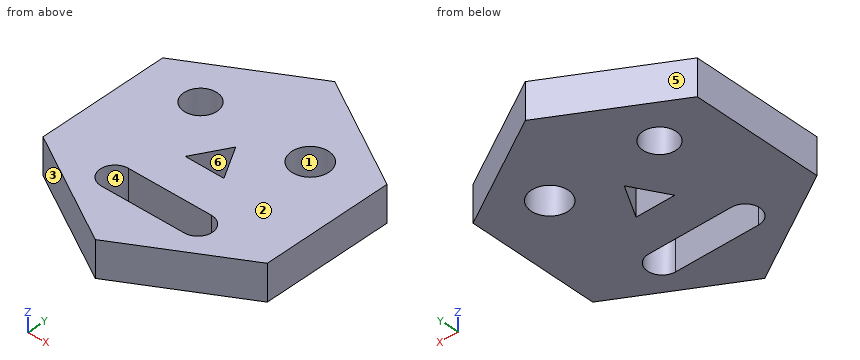
from build123d import *

# Parameters (mm, degrees)
SKETCH_R   = 4.618848
SKETCH_R_2 = 5.157962
PAD_DEPTH  = 10


with BuildPart() as part:
    # Sketch → Pad (new body)
    with BuildSketch(Plane.XY):
        Polygon((96.723577, 31.138338), (96.674117, 67.116094), (65.491737, 85.062138), (34.358817, 67.030427), (34.408277, 31.052671), (65.590657, 13.106627), align=None)
        with Locations((50.045269, 61.452663)):
            Circle(SKETCH_R, mode=Mode.SUBTRACT)
        with Locations((80.082733, 61.98597)):
            Circle(SKETCH_R_2, mode=Mode.SUBTRACT)
        with BuildLine():
            ThreePointArc((54.325382, 35.182339), (50.269895, 31.126852), (54.325382, 27.071365))
            Line((54.325382, 27.071365), (77.411652, 27.071365))
            ThreePointArc((77.411652, 27.071365), (81.467139, 31.126852), (77.411652, 35.182339))
            Line((54.325382, 35.182339), (77.411652, 35.182339))
        make_face(mode=Mode.SUBTRACT)
        Polygon((65.553779, 55.296537), (60.155022, 45.989201), (70.91479, 45.967409), align=None, mode=Mode.SUBTRACT)
    extrude(amount=PAD_DEPTH)


solid = part.part
Input: part model. Units: mm. Frame: model coordinates. Face numbers are marked on the shaded views. A direction names the side the tool comes from. Give positions to 0.01 mm unless a question says otherwise; leave off trailing zeros. Loops run counter-clockwise (first coordinate to the right, second up) from the corner with the lowest first, then second, coordinate; pieces in that order, holes last. Notation, with made-up numbers: (14.25, 69.5) -> (70.25, 69.5) arc R19 ccw to (70.25, 82.5) -> close; hole circle Ø5 at (-34.75, 71.25). An arc over 180 degrees is marked (long way). Answer as a JSON object with one key per item and string values. Group by question number.
Item 1: Cut plane D-D, the plane y = 58. Return the cut outline in (x, z), and give its area (3 significant figures).
Item 2: Cut plane B-B, the plane x = 58. Return the cut outline in (y, z).
Item 3: Line query: probe 1 along Y at (x, z) = (80, 9); probe 2 along Y at (x, z) = (60.5, 3); probe 3 along X at (y, z) = (55.5, 1.5). Output: solid intervals per line, ascending.
Item 4: Pull-direction query (Y, two-part tool) for the marked faces 1, 2, 3 and 4; classes: released by +Y, released by -Y, zero draft, split by the parting line, or undercut.
Item 5: Reachability of the marked faces 5 and 6 from +Z, -Z, +X, -X, +Y, -Y: full face, straight path, thin tool, end or side. Return the list, or none.
Item 6: Cut plane A-A, the plane y = 47.5. Return the cut outline in (x, z), and give its area (3 significant figures).
Item 7: Pin query (flat end, axial travel): P1, Ø5, axis at y = 60, z = 8, coming from the +X side; P2, Ø3, axis at x = 62, z = 2, coming from the -Y side; P3, Ø4, axis at y = 35.5, z = 6.5, coming from the -X side. Return the tip coordinate at first contact, or that it passes through.
Item 8: Cut plane C-C, the plane z = 8. Return the cut outline in (x, y), and give its area (3 significant figures).
Checks:
{
 "1": {"outline": "(34.37, 0) -> (46.98, 0) -> (46.98, 10) -> (34.37, 10) -> close; (53.11, 0) -> (76.81, 0) -> (76.81, 10) -> (53.11, 10) -> close; (83.36, 0) -> (96.69, 0) -> (96.69, 10) -> (83.36, 10) -> close", "area": "496 mm²"},
 "2": {"outline": "(17.48, 0) -> (27.07, 0) -> (27.07, 10) -> (17.48, 10) -> close; (35.18, 0) -> (80.72, 0) -> (80.72, 10) -> (35.18, 10) -> close"},
 "3": {"probe 1": "y = 21.45 to 28, 34.25 to 56.83, 67.14 to 76.71", "probe 2": "y = 16.04 to 27.07, 35.18 to 45.99, 46.58 to 82.17", "probe 3": "x = 34.37 to 96.69"},
 "4": {"face 1": "undercut", "face 2": "zero draft", "face 3": "released by -Y", "face 4": "undercut"},
 "5": {"face 5": "+Z, -Z, -X, +Y", "face 6": "+Z, -Z"},
 "6": {"outline": "(34.39, 0) -> (61.03, 0) -> (61.03, 10) -> (34.39, 10) -> close; (70.03, 0) -> (96.7, 0) -> (96.7, 10) -> (70.03, 10) -> close", "area": "533 mm²"},
 "7": {"P1": "stops at x = 96.69", "P2": "stops at y = 14.31", "P3": "stops at x = 34.4"},
 "8": {"outline": "(34.36, 67.03) -> (34.41, 31.05) -> (65.59, 13.11) -> (96.72, 31.14) -> (96.67, 67.12) -> (65.49, 85.06) -> close; hole circle Ø9.24 at (50.05, 61.45); hole (54.33, 27.07) -> (77.41, 27.07) arc R4.06 ccw to (77.41, 35.18) -> (54.33, 35.18) arc R4.06 ccw to start; hole (60.16, 45.99) -> (70.91, 45.97) -> (65.55, 55.3) -> close; hole circle Ø10.32 at (80.08, 61.99)", "area": "2,920 mm²"}
}
